from build123d import *

# Parameters (mm, degrees)
BOSS_EXTRUDE1_DEPTH          = 3.175
SKETCH2_R                    = 14.2875
CUT_EXTRUDE1_DEPTH           = 131.459778054
F_10_0_1935_DIAMETER_HOLE2_D = 4.9149


with BuildPart() as part:
    # Sketch1 → Boss-Extrude1 (new, symmetric)
    with BuildSketch(Plane.XY):
        Polygon((-76.2, 29.162153383), (-127, -21.637846617), (127, -21.637846617), (76.2, 29.162153383), align=None)
    extrude(amount=BOSS_EXTRUDE1_DEPTH, both=True)

    # Sketch2 → Cut-Extrude1 (cut, through all)
    with BuildSketch(Plane.XY.offset(3.175)):
        with Locations((-36.107951031, -2.587846617)):
            Circle(SKETCH2_R)
    extrude(amount=-CUT_EXTRUDE1_DEPTH, mode=Mode.SUBTRACT)

    # #10 (0.1935) Diameter Hole2 (through all)
    with Locations(Plane(origin=(62.861792847, 24.539848294, 3.175), x_dir=(1, 0, 0), z_dir=(0, 0, 1))):
        with Locations((0, 0), (35.921024485, -35.921024485), (-152.664354058, -26.940768364)):
            Hole(F_10_0_1935_DIAMETER_HOLE2_D / 2)


solid = part.part
Verification items for the finished model (mm, model axes). Coordinates: 2 decimals unless noted, no trailing zeros. Order: outer loops, then holes, each group sorted by start corner. A loop starts at its lowest first (then second) coordinate and runs counter-clockwise, first axis right, second up. Notation, with made-up numbers: (-33.75, 0.5) -> (-29.75, 0.5) arc R12 ccw to (-29.75, 11.5) -> close; hole circle Ø9 at (-16.75, 59.25). An arc over 180 degrees is marked (long way). Put each result on its own line as item: value. Start each with the question number.
1. Material ranges on L1, parallel to X at y = -12, z = 2.25; L2, parallel to X at y = -2, z = 0; L3, parallel to Y at x = -25, z = -1.25, recorded low to high. Write a range as [from, to].
2. Cross-section at B-B, the plane y = 16.5. Record the boundary of the cut face in (x, z) (3 decimals), then the cut area to 3 significant figures.
3. Cross-section at A-A, the plane z = -0.25. Record the boundary of the cut face in (x, y) (1 decimal).
4. Go/stop test with a flat-tipped pin: pin 1 Ø4 at (x, y) = (98.78, -11.38) entering from -Z. Record where the tip stops, or that it passes through.
5. Mould release check, pull along X, two halves, no side actions. Record for faces 1 (the flat face through (-2, -21.638, 0)), 2 (the flat face through (-101.24, 4.12, 0.04)), 3 (the cylindrical face through (65.317, 24.648, -0.044)): released by +X, released by -X, zero draft, split by the parting line, or undercut.
Computed:
1. L1: [-117.36, -46.86], [-25.36, 96.4], [101.16, 117.36]
1. L2: [-107.36, -92.23], [-87.38, -50.38], [-21.83, 107.36]
1. L3: [-21.64, -11.57], [6.4, 29.16]
2. outline: (-88.862, -3.175) -> (88.862, -3.175) -> (88.862, 3.175) -> (-88.862, 3.175) -> close
2. area: 1,130 mm2
3. outline: (-127, -21.6) -> (127, -21.6) -> (76.2, 29.2) -> (-76.2, 29.2) -> close; hole circle Ø4.9 at (-89.8, -2.4); hole circle Ø28.6 at (-36.1, -2.6); hole circle Ø4.9 at (62.9, 24.5); hole circle Ø4.9 at (98.8, -11.4)
4. pin 1: through
5. face 1: zero draft
5. face 2: released by -X
5. face 3: undercut
